Design review of the part shown in the three views and the two pictorial views. Dimensions are in mm from the part's minimum x, y and z. A direction names the side the tool comes from. Give positions to 0.01 mm unless a question says otherwise; leave off trailing zeros. Write each loop counter-clockwise with the first axis right and the second up, starting at its lowest first coordinate (ties: lowest second). Pieces come first, ordered by that corner, then holes. Notation, with made-up numbers: M 50.25,33 L 92.25,33 A21 cw 92.25,51 Z; hole C -10.75,70 d11. An arc over 180 degrees is marked long. Write item = value, one per line.
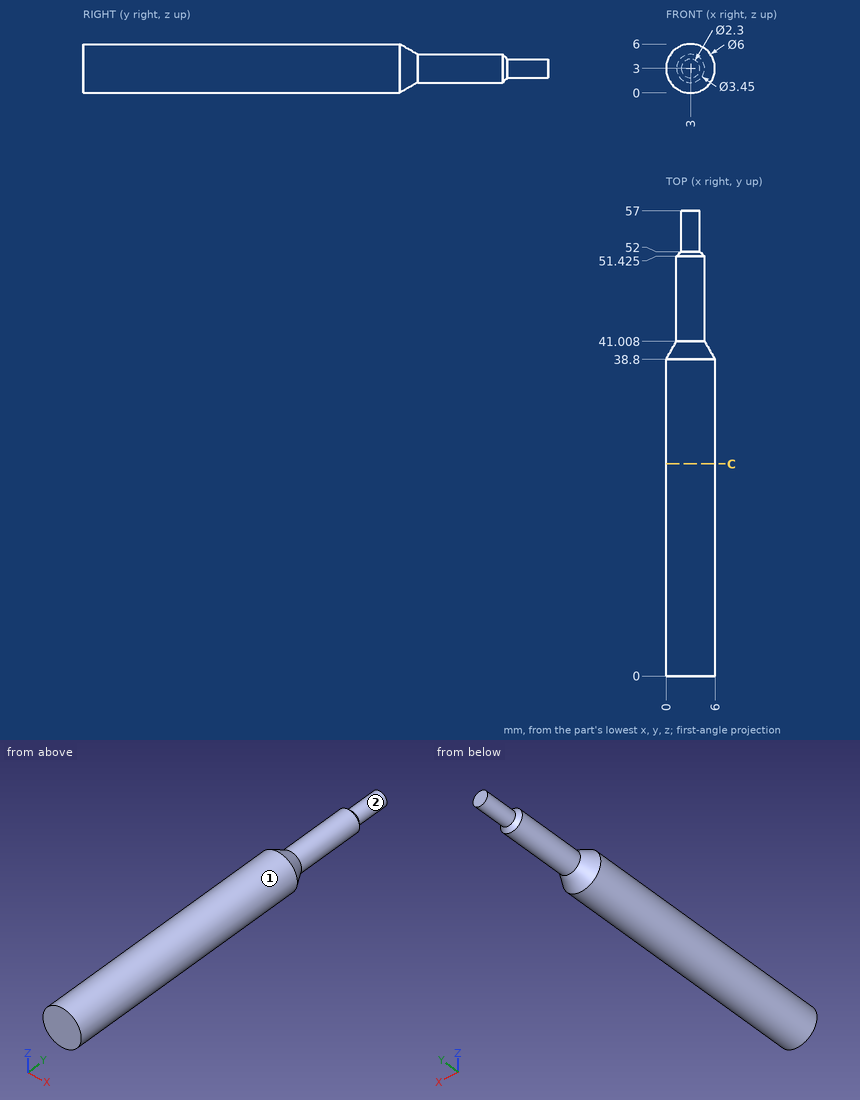
1. We need section C-C, the plane y = 26. Write out the cut boundary in (x, z), then the cut area to 3 significant figures.
Responses:
outline = C 3,3 d6
area = 28.3 mm2
2. Insertion check: P1, Ø1, axis at y = 25, z = 4.5, coming from the +X side; P2, Ø2, axis at y = 47.5, z = 2.5, coming from the +X side (3 decimals). Each pin has a flat end and moves straight along its axis. Give the tip position at first contact, or say it passes through.
Responses:
P1 = 5.83
P2 = 4.725
3. Machinability: for the marked faces 1 and 2, which of the approach directions +Z, -Z, +X, -X, +Y, -Y give a long, thin tool a straight path to every point of the face, cutting with its end or side? Answer none if there is none.
Responses:
face_1 = +Y, -Y
face_2 = +Y
4. For line 1 along Z through (x, y) = (2.8, 31); line 2 along X through (y, z) = (18, 2.85); line 3 along Y through (x, z) = (0.85, 4), list the stretches that pass through material, from the lowest coordinate up. Write a range as from..to.
Responses:
line_1 = 0.01..5.99
line_2 = 0..6
line_3 = 0..39.89
